```python
from build123d import *

# Parameters (mm, degrees)
FILLET1_R  = 0.8
SKETCH2_W  = 5.5
SKETCH2_H  = 0.8
SLOT_DEPTH = 0.85


with BuildPart() as part:
    # BodySke → Base-Revolve (revolve)
    with BuildSketch(Plane.XY, mode=Mode.PRIVATE) as base_revolve_sk:
        Polygon((0, 0), (0, 2.75), (0.4, 2.75), (1.65, 1.5), (10, 1.5), (10, 0), align=None)
    revolve(base_revolve_sk.sketch.rotate(Axis((-6.35, 0, 0), (1, 0, 0)), 90), axis=Axis((-6.35, 0, 0), (1, 0, 0)))  # turned: the seam where the file's is

    # Fillet1
    fillet1_edges = [part.edges().sort_by_distance(p)[0] for p in [
        (1.65, 0, -1.5),
    ]]
    fillet(fillet1_edges, radius=FILLET1_R)

    # Sketch2 → Slot (cut)
    with BuildSketch(Plane.ZY):
        Rectangle(SKETCH2_W, SKETCH2_H)
    extrude(amount=-SLOT_DEPTH, mode=Mode.SUBTRACT)


solid = part.part
```
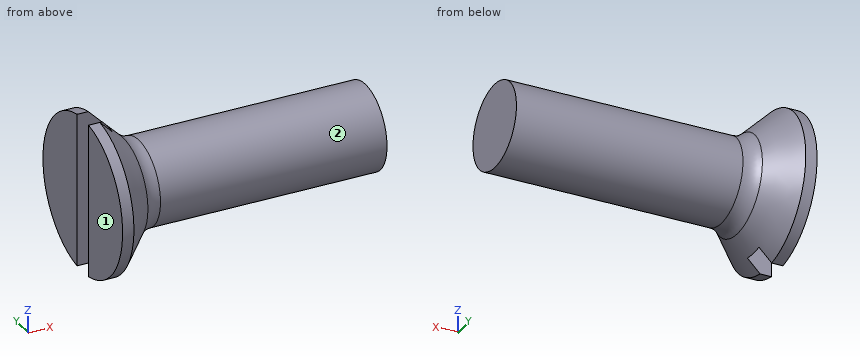
Part model, mm, in its own coordinate system. Face numbers are marked on the shaded views. A direction names the side the tool comes from. Round coordinates to 2 decimals unless told otherwise and drop trailing zeros. Loops run counter-clockwise (first coordinate to the right, second up) from the corner with the lowest first, then second, coordinate; pieces in that order, holes last.
1. Drill centre lines: line 1 along X through (y, z) = (-1.9, -0.65); line 2 along X through (y, z) = (1.3, 1.8); line 3 along Y through (x, z) = (4.25, -0.15). Where is each one in solid material? Low to high.
Solutions:
line 1: x = 0 to 1.14
line 2: x = 0 to 0.93
line 3: y = -1.49 to 1.49
2. Flat gauge pin, fed straight in: pin 1 (1.5 mm diameter, centred on x = 3.5, y = 1, fed in from +Z). Where does the tip first touch, or does it go through?
Solutions:
pin 1: stops at z = 1.48
3. 3-axis set-ups, long thin cutter, end or side, ignore diameter. For the marked faces 1 and 2: which of +Z, -Z, +X, -X, +Y, -Y reach the whole face in a straight line?
Solutions:
face 1: +Z, -Z, -X, +Y, -Y
face 2: +X
4. Slice it at A-A (x = 2.25). Give the cut face in (y, z).
Solutions:
outline: circle Ø3 at (0, 0)
